```python
from build123d import *

# Parameters (mm, degrees)
SKETCH_1_R             = 3.5
SKETCH_1_R_2           = 1.65
EXTRUDE_1_DEPTH        = 25
HOLE_WIZARD_M4_1_D     = 3.3
HOLE_WIZARD_M4_1_DEPTH = 10
HOLE_WIZARD_M4_1_TIP   = 0.991420021
HOLE_WIZARD_M4_2_D     = 3.3
HOLE_WIZARD_M4_2_DEPTH = 10
HOLE_WIZARD_M4_2_TIP   = 0.991420021
CHAMFER_1_SIZE         = 0.3


with BuildPart() as part:
    # 스케치1 → 보스-돌출1 (new body)
    # profile 1 of 2: a face of its own
    with BuildSketch(Plane(origin=(0, 0, 0), x_dir=(1, 0, 0), z_dir=(0, 1, 0))):
        with Locations(Location((0, 0, 0), (0, 0, 270))):
            Circle(SKETCH_1_R)
        Circle(SKETCH_1_R_2, mode=Mode.SUBTRACT)
    # profile 2 of 2: a face of its own
    with BuildSketch(Plane(origin=(0, 0, 0), x_dir=(1, 0, 0), z_dir=(0, 1, 0))):
        Circle(SKETCH_1_R_2)
    extrude(amount=EXTRUDE_1_DEPTH)

    # M4 탭을 위한 탭 드릴1
    with Locations(Plane(origin=(0, 0, 0), x_dir=(-1, 0, 0), z_dir=(0, -1, 0))):
        with Locations((0, 0)):
            Hole(HOLE_WIZARD_M4_1_D / 2, depth=HOLE_WIZARD_M4_1_DEPTH)
            with Locations((0, 0, -(HOLE_WIZARD_M4_1_DEPTH + HOLE_WIZARD_M4_1_TIP / 2))):  # 118° drill point
                Cone(0, HOLE_WIZARD_M4_1_D / 2, HOLE_WIZARD_M4_1_TIP, mode=Mode.SUBTRACT)

    # M4 탭을 위한 탭 드릴2
    with Locations(Plane(origin=(0, 25, 0), x_dir=(1, 0, 0), z_dir=(0, 1, 0))):
        with Locations((0, 0)):
            Hole(HOLE_WIZARD_M4_2_D / 2, depth=HOLE_WIZARD_M4_2_DEPTH)
            with Locations((0, 0, -(HOLE_WIZARD_M4_2_DEPTH + HOLE_WIZARD_M4_2_TIP / 2))):  # 118° drill point
                Cone(0, HOLE_WIZARD_M4_2_D / 2, HOLE_WIZARD_M4_2_TIP, mode=Mode.SUBTRACT)

    # 모따기1
    chamfer_1_edges = [part.edges().sort_by_distance(p)[0] for p in [
        (1.65, 25, 0),
        (0, 0, -3.5),
        (0, 25, -3.5),
        (-1.65, 0, 0),
    ]]
    chamfer(chamfer_1_edges, length=CHAMFER_1_SIZE)


solid = part.part
```
The model under review builds one solid part; all positions refer to its coordinate system, in mm. A direction names the side the tool comes from. Round coordinates to 2 decimals unless told otherwise and drop trailing zeros. Loops run counter-clockwise (first coordinate to the right, second up) from the corner with the lowest first, then second, coordinate; pieces in that order, holes last. Notation, with made-up numbers: (-39, 45.25) -> (-19, 45.25) arc R33 cw to (-19, 84.25) -> close; hole circle Ø11 at (48, -30). An arc over 180 degrees is marked (long way). Answer as a JSON object with one key per item and string values. Group by question number.
1) For line 1 (X direction, y = 6.25, z = 0); line 2 (X direction, y = 1.25, z = -0.75); line 3 (Z direction, x = 2, y = 19), list the stretches that pass through material, from the lowest coordinate up. Write a range as [from, to].
2) We need section A-A on y = 9. Write out the cut boundary in (x, z), then the cut area to 3 significant figures.
3) For faces 1 (the face through (0, 25, 2.1)), 2 (the face through (1.216, 19.782, -1.115)), list the 3-axis set-ups (+Z, -Z, +X, -X, +Y, -Y) from which the entire face can be reached by the end or side of a thin tool; tool diameter is ignored.
4) Mouldability with a two-part tool opening along Z and no side actions: class faces 3 (the face through (-3.417, 12.329, -0.759)), 4 (the face through (0, 0, 2.1)), 5 (the face through (-1.216, 5.218, -1.115)) as released by +Z, released by -Z, zero draft, split by the parting line, or undercut.
5) For pin 1 Ø2 at (x, y) = (-2.5, 9) entering from -Z; pin 2 Ø3 at (x, y) = (2.5, 3) entering from +Z; pin 3 Ø4 at (x, y) = (-2.5, 3.5) entering from -Z, all flat-tipped, find the tip position at first contact; note any pin that passes through.
Result set:
{
 "1": {"line 1": "[-3.5, -1.65], [1.65, 3.5]", "line 2": "[-3.42, -1.47], [1.47, 3.42]", "line 3": "[-2.87, 2.87]"},
 "2": {"outline": "circle Ø7 at (0, 0); hole circle Ø3.3 at (0, 0)", "area": "29.9 mm²"},
 "3": {"face 1": "+Z, -Z, +X, -X, +Y", "face 2": "+Y"},
 "4": {"face 3": "split by the parting line", "face 4": "zero draft", "face 5": "undercut"},
 "5": {"pin 1": "z = -3.16", "pin 2": "z = 3.35", "pin 3": "z = -3.46"}
}
